Geometry: final body of the model. Coordinates: model frame, mm. Round coordinates to 2 decimals unless told otherwise and drop trailing zeros. Write each loop counter-clockwise with the first axis right and the second up, starting at its lowest first coordinate (ties: lowest second). Pieces come first, ordered by that corner, then holes. Notation, with made-up numbers: (36, -9.75) - (77, -9.75) arc R25 ccw to (77, 29.25) - close; hole circle Ø3 at (57, 82). An arc over 180 degrees is marked (long way). Write each question's results on one line, items separated by ' | '.
from build123d import *

# Parameters (mm, degrees)
SKETCH1_W           = 40
SKETCH1_H           = 40
SKETCH1_R           = 1.5
SKETCH1_R_2         = 2.2479
SKETCH1_H_2         = 47.5
SKETCH1_W_2         = 47.5
BOSS_EXTRUDE1_DEPTH = 3.175
SKETCH1_6_R         = 1.5
BOSS_EXTRUDE2_DEPTH = 1.5875


with BuildPart() as part:
    # Sketch1 → Boss-Extrude1 (new body)
    # profile 1 of 5: a face of its own
    with BuildSketch(Plane.XY):
        Rectangle(SKETCH1_W, SKETCH1_H)
        with Locations((-15, -18)):
            Circle(SKETCH1_R, mode=Mode.SUBTRACT)
        with Locations((-18, -15)):
            Circle(SKETCH1_R, mode=Mode.SUBTRACT)
        with Locations((-10.253048327, -10.253048327)):
            Circle(SKETCH1_R_2, mode=Mode.SUBTRACT)
        with Locations((15, -18)):
            Circle(SKETCH1_R, mode=Mode.SUBTRACT)
        with Locations((18, -15)):
            Circle(SKETCH1_R, mode=Mode.SUBTRACT)
        with Locations((-18, 15)):
            Circle(SKETCH1_R, mode=Mode.SUBTRACT)
        with Locations((-10.253048327, 10.253048327)):
            Circle(SKETCH1_R_2, mode=Mode.SUBTRACT)
        with Locations((-15, 18)):
            Circle(SKETCH1_R, mode=Mode.SUBTRACT)
        Circle(SKETCH1_R_2, mode=Mode.SUBTRACT)
        with Locations((18, 15)):
            Circle(SKETCH1_R, mode=Mode.SUBTRACT)
        with Locations((15, 18)):
            Circle(SKETCH1_R, mode=Mode.SUBTRACT)
    # profile 2 of 5: a face of its own
    with BuildSketch(Plane.XY):
        with Locations((0, 43.75)):
            Rectangle(SKETCH1_W, SKETCH1_H_2)
        with Locations((-15, 27.9)):
            Circle(SKETCH1_R, mode=Mode.SUBTRACT)
        with Locations((-15, 37.8)):
            Circle(SKETCH1_R, mode=Mode.SUBTRACT)
        with Locations((-15, 47.7)):
            Circle(SKETCH1_R, mode=Mode.SUBTRACT)
        with Locations((-15, 57.6)):
            Circle(SKETCH1_R, mode=Mode.SUBTRACT)
        with Locations((-5, 57.6)):
            Circle(SKETCH1_R, mode=Mode.SUBTRACT)
        with Locations((15, 27.9)):
            Circle(SKETCH1_R, mode=Mode.SUBTRACT)
        with Locations((15, 37.8)):
            Circle(SKETCH1_R, mode=Mode.SUBTRACT)
        with Locations((15, 47.7)):
            Circle(SKETCH1_R, mode=Mode.SUBTRACT)
        with Locations((5, 57.6)):
            Circle(SKETCH1_R, mode=Mode.SUBTRACT)
        with Locations((15, 57.6)):
            Circle(SKETCH1_R, mode=Mode.SUBTRACT)
    # profile 3 of 5: a face of its own
    with BuildSketch(Plane.XY):
        with Locations((43.75, 0)):
            Rectangle(SKETCH1_W_2, SKETCH1_H)
        with Locations((27.9, -15)):
            Circle(SKETCH1_R, mode=Mode.SUBTRACT)
        with Locations((37.8, -15)):
            Circle(SKETCH1_R, mode=Mode.SUBTRACT)
        with Locations((47.7, -15)):
            Circle(SKETCH1_R, mode=Mode.SUBTRACT)
        with Locations((57.6, -15)):
            Circle(SKETCH1_R, mode=Mode.SUBTRACT)
        with Locations((57.6, -5)):
            Circle(SKETCH1_R, mode=Mode.SUBTRACT)
        with Locations((27.9, 15)):
            Circle(SKETCH1_R, mode=Mode.SUBTRACT)
        with Locations((48.94, 0)):
            Circle(SKETCH1_R_2, mode=Mode.SUBTRACT)
        with Locations((37.8, 15)):
            Circle(SKETCH1_R, mode=Mode.SUBTRACT)
        with Locations((47.7, 15)):
            Circle(SKETCH1_R, mode=Mode.SUBTRACT)
        with Locations((57.6, 5)):
            Circle(SKETCH1_R, mode=Mode.SUBTRACT)
        with Locations((57.6, 15)):
            Circle(SKETCH1_R, mode=Mode.SUBTRACT)
    # profile 4 of 5: a face of its own
    with BuildSketch(Plane.XY):
        with Locations((-43.75, 0)):
            Rectangle(SKETCH1_W_2, SKETCH1_H)
        with Locations((-57.6, -15)):
            Circle(SKETCH1_R, mode=Mode.SUBTRACT)
        with Locations((-57.6, -5)):
            Circle(SKETCH1_R, mode=Mode.SUBTRACT)
        with Locations((-47.7, -15)):
            Circle(SKETCH1_R, mode=Mode.SUBTRACT)
        with Locations((-37.8, -15)):
            Circle(SKETCH1_R, mode=Mode.SUBTRACT)
        with Locations((-27.9, -15)):
            Circle(SKETCH1_R, mode=Mode.SUBTRACT)
        with Locations((-57.6, 5)):
            Circle(SKETCH1_R, mode=Mode.SUBTRACT)
        with Locations((-57.6, 15)):
            Circle(SKETCH1_R, mode=Mode.SUBTRACT)
        with Locations((-47.7, 15)):
            Circle(SKETCH1_R, mode=Mode.SUBTRACT)
        with Locations((-37.8, 15)):
            Circle(SKETCH1_R, mode=Mode.SUBTRACT)
        with Locations((-27.9, 15)):
            Circle(SKETCH1_R, mode=Mode.SUBTRACT)
    # profile 5 of 5: a face of its own
    with BuildSketch(Plane.XY):
        with Locations((0, -43.75)):
            Rectangle(SKETCH1_W, SKETCH1_H_2)
        with Locations((-15, -57.6)):
            Circle(SKETCH1_R, mode=Mode.SUBTRACT)
        with Locations((-5, -57.6)):
            Circle(SKETCH1_R, mode=Mode.SUBTRACT)
        with Locations((-15, -47.7)):
            Circle(SKETCH1_R, mode=Mode.SUBTRACT)
        with Locations((-15, -37.8)):
            Circle(SKETCH1_R, mode=Mode.SUBTRACT)
        with Locations((-15, -27.9)):
            Circle(SKETCH1_R, mode=Mode.SUBTRACT)
        with Locations((5, -57.6)):
            Circle(SKETCH1_R, mode=Mode.SUBTRACT)
        with Locations((15, -57.6)):
            Circle(SKETCH1_R, mode=Mode.SUBTRACT)
        with Locations((15, -47.7)):
            Circle(SKETCH1_R, mode=Mode.SUBTRACT)
        with Locations((15, -37.8)):
            Circle(SKETCH1_R, mode=Mode.SUBTRACT)
        with Locations((15, -27.9)):
            Circle(SKETCH1_R, mode=Mode.SUBTRACT)
    extrude(amount=BOSS_EXTRUDE1_DEPTH)

    # Sketch1_6 → Boss-Extrude2 (add)
    with BuildSketch(Plane.XY):
        with Locations((18, 15)):
            Circle(SKETCH1_6_R)
        with Locations((15, 18)):
            Circle(SKETCH1_6_R)
        with Locations((27.9, 15)):
            Circle(SKETCH1_6_R)
        with Locations((37.8, 15)):
            Circle(SKETCH1_6_R)
        with Locations((47.7, 15)):
            Circle(SKETCH1_6_R)
        with Locations((57.6, 5)):
            Circle(SKETCH1_6_R)
        with Locations((57.6, -5)):
            Circle(SKETCH1_6_R)
        with Locations((57.6, -15)):
            Circle(SKETCH1_6_R)
        with Locations((47.7, -15)):
            Circle(SKETCH1_6_R)
        with Locations((37.8, -15)):
            Circle(SKETCH1_6_R)
        with Locations((18, -15)):
            Circle(SKETCH1_6_R)
        with Locations((15, -18)):
            Circle(SKETCH1_6_R)
        with Locations((27.9, -15)):
            Circle(SKETCH1_6_R)
        with Locations((15, -27.9)):
            Circle(SKETCH1_6_R)
        with Locations((15, -47.7)):
            Circle(SKETCH1_6_R)
        with Locations((15, -37.8)):
            Circle(SKETCH1_6_R)
        with Locations((15, -57.6)):
            Circle(SKETCH1_6_R)
        with Locations((5, -57.6)):
            Circle(SKETCH1_6_R)
        with Locations((-5, -57.6)):
            Circle(SKETCH1_6_R)
        with Locations((-15, -57.6)):
            Circle(SKETCH1_6_R)
        with Locations((-15, -47.7)):
            Circle(SKETCH1_6_R)
        with Locations((-15, -37.8)):
            Circle(SKETCH1_6_R)
        with Locations((-15, -27.9)):
            Circle(SKETCH1_6_R)
        with Locations((-15, -18)):
            Circle(SKETCH1_6_R)
        with Locations((-18, -15)):
            Circle(SKETCH1_6_R)
        with Locations((-27.9, -15)):
            Circle(SKETCH1_6_R)
        with Locations((-37.8, -15)):
            Circle(SKETCH1_6_R)
        with Locations((-47.7, -15)):
            Circle(SKETCH1_6_R)
        with Locations((-57.6, -15)):
            Circle(SKETCH1_6_R)
        with Locations((-57.6, -5)):
            Circle(SKETCH1_6_R)
        with Locations((-57.6, 15)):
            Circle(SKETCH1_6_R)
        with Locations((-57.6, 5)):
            Circle(SKETCH1_6_R)
        with Locations((-47.7, 15)):
            Circle(SKETCH1_6_R)
        with Locations((-37.8, 15)):
            Circle(SKETCH1_6_R)
        with Locations((-15, 18)):
            Circle(SKETCH1_6_R)
        with Locations((-18, 15)):
            Circle(SKETCH1_6_R)
        with Locations((-27.9, 15)):
            Circle(SKETCH1_6_R)
        with Locations((-15, 27.9)):
            Circle(SKETCH1_6_R)
        with Locations((-15, 47.7)):
            Circle(SKETCH1_6_R)
        with Locations((-15, 37.8)):
            Circle(SKETCH1_6_R)
        with Locations((-15, 57.6)):
            Circle(SKETCH1_6_R)
        with Locations((-5, 57.6)):
            Circle(SKETCH1_6_R)
        with Locations((5, 57.6)):
            Circle(SKETCH1_6_R)
        with Locations((15, 57.6)):
            Circle(SKETCH1_6_R)
        with Locations((15, 47.7)):
            Circle(SKETCH1_6_R)
        with Locations((15, 37.8)):
            Circle(SKETCH1_6_R)
        with Locations((15, 27.9)):
            Circle(SKETCH1_6_R)
        with Locations((57.6, 15)):
            Circle(SKETCH1_6_R)
    extrude(amount=BOSS_EXTRUDE2_DEPTH)


solid = part.part
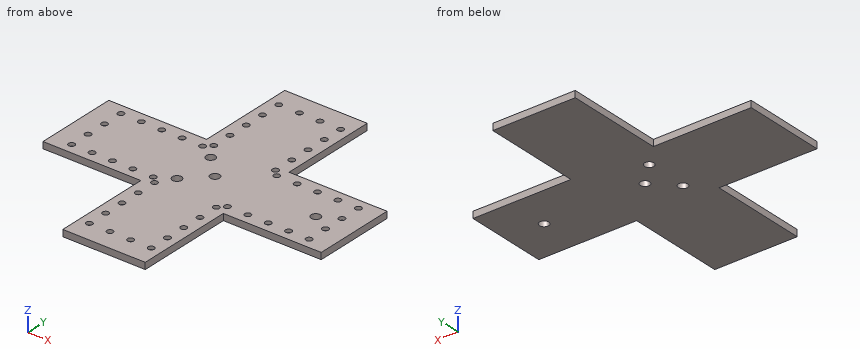
Q1. Section query B-B, the plane y = -54. Return loops of the section in (x, z) (3 decimals).
Answer block:
outline: (-20, 0) - (20, 0) - (20, 3.175) - (-20, 3.175) - close
Q2. Section query A-A, the plane z = 0.95. Return loops of the section in (x, y).
Answer block:
outline: (-67.5, -20) - (-20, -20) - (-20, -67.5) - (20, -67.5) - (20, -20) - (67.5, -20) - (67.5, 20) - (20, 20) - (20, 67.5) - (-20, 67.5) - (-20, 20) - (-67.5, 20) - close; hole circle Ø4.5 at (-10.25, -10.25); hole circle Ø4.5 at (-10.25, 10.25); hole circle Ø4.5 at (0, 0); hole circle Ø4.5 at (48.94, 0)
Q3. Pin query (flat end, axial travel): pin 1 (0.9 mm diameter, centred on x = 14.5, y = -17.5, fed in from +Z); pin 2 (1 mm diameter, centred on y = -43, z = 1, fed in from +X); pin 3 (3.5 mm diameter, centred on x = 4.5, y = 57, fed in from +Z) (3 decimals); pin 4 (1.5 mm diameter, centred on x = 51.5, z = 2.5, fed in from +Y). Return the tip coordinate at first contact, or that it passes through.
Answer block:
pin 1: z = 1.59 | pin 2: x = 20 | pin 3: z = 3.175 | pin 4: y = 20
Q4. Ray query, line 1 along Y through (x, z) = (-18, 2.4); line 2 along Y through (x, z) = (57.6, 2.55); line 3 along Y through (x, z) = (38, 2.65). Return the intervals inside material, ascending.
Answer block:
line 1: -67.5 to -16.5, -13.5 to 13.5, 16.5 to 67.5 | line 2: -20 to -16.5, -13.5 to -6.5, -3.5 to 3.5, 6.5 to 13.5, 16.5 to 20 | line 3: -20 to -16.49, -13.51 to 13.51, 16.49 to 20
